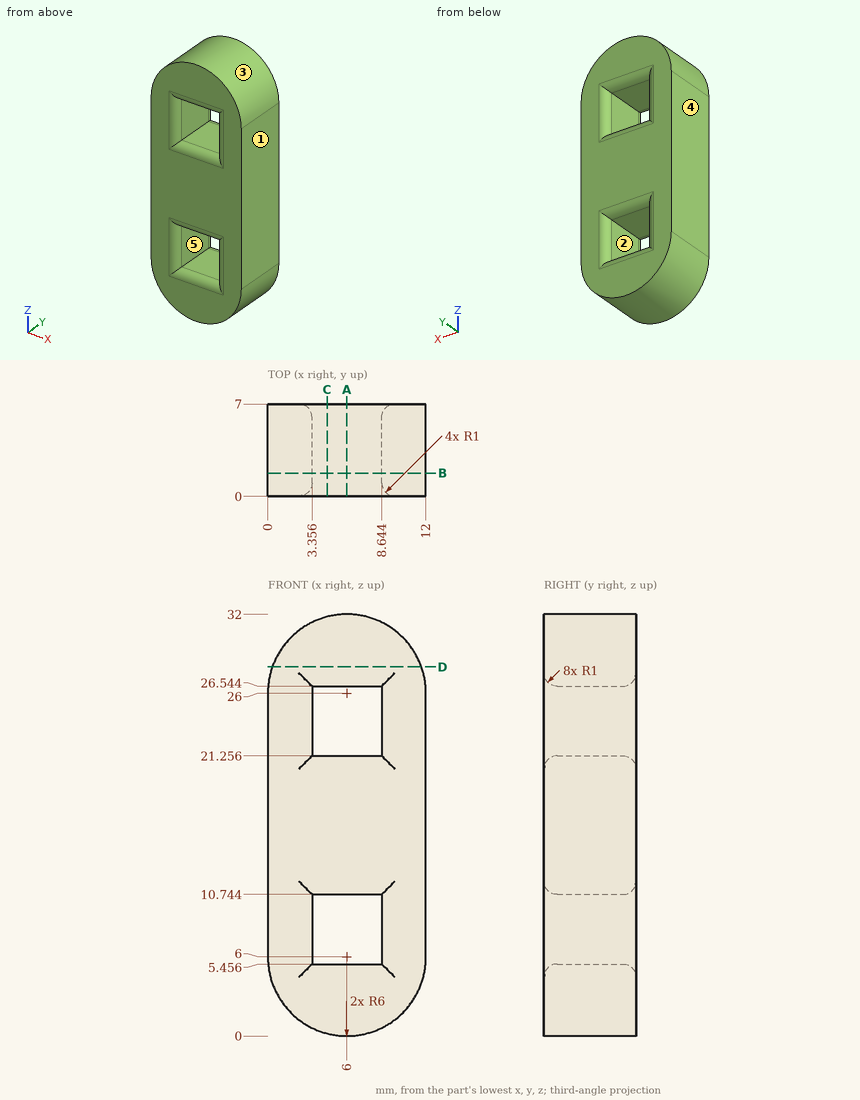
Source: three-view drawing plus pictorial views. Frame: mm from the lowest corner of the part. A direction names the side the tool comes from. Coordinates: 2 decimals unless noted, no trailing zeros. Loops run counter-clockwise (first coordinate to the right, second up) from the corner with the lowest first, then second, coordinate; pieces in that order, holes last. Notation, with made-up numbers: (-30.5, -36.75) -> (-11.5, -36.75) arc R21 ccw to (-11.5, -9.75) -> close; hole circle Ø1 at (-9, 41). An arc over 180 degrees is marked (long way). Answer in a Markdown table with one row per item. Add a question column.
Q1. Section C-C on x = 4.5. Return the cut outline in (y, z).
Q2. Section A-A on x = 6. Return the cut outline in (y, z), and give its area (3 significant figures).
Q3. Section B-B on y = 1.75. Return the cut outline in (x, z), and give its area (3 significant figures).
Q4. Ray query, line 1 along Z through (x, y) = (6.25, 3.25); line 2 along X through (y, z) = (6, 8); line 3 along Z through (x, y) = (6.25, 6.5). Return the intervals inside material, ascending.
Q5. Pull-direction query (Z, two-part tool) for the marked faces 1, 2 and 3; classes: pulls with the +Z half, pulls with the -Z half, needs draft (parallel to the pull), parting line crosses it, or undercut.
Q6. Section D-D on z = 28. Return the cut outline in (x, y), and give its area (3 significant figures).
Q7. Contact query for flat-ended pins moving along their axis: pin 1 Ø1 at (x, y) = (10.5, 1) entering from -Z; pin 2 Ø1 at (y, z) = (4.5, 4) entering from +X; pin 3 Ø2 at (x, z) = (8, 22) entering from -Y (3 decimals). Output: stop coordinate, or through.
Q8. Reachability of the marked faces 4 and 5 from +Z, -Z, +X, -X, +Y, -Y: full face, straight path, thin tool, end or side. Return the list, or none.
Computed values:
| question | item | result |
|---|---|---|
| 1 | outline | (0, 0.19) -> (7, 0.19) -> (7, 4.46) arc R1 ccw to (6, 5.46) -> (1, 5.46) arc R1 ccw to (0, 4.46) -> close; (0, 11.74) arc R1 ccw to (1, 10.74) -> (6, 10.74) arc R1 ccw to (7, 11.74) -> (7, 20.26) arc R1 ccw to (6, 21.26) -> (1, 21.26) arc R1 ccw to (0, 20.26) -> close; (0, 27.54) arc R1 ccw to (1, 26.54) -> (6, 26.54) arc R1 ccw to (7, 27.54) -> (7, 31.81) -> (0, 31.81) -> close |
| 2 | outline | (0, 0) -> (7, 0) -> (7, 4.46) arc R1 ccw to (6, 5.46) -> (1, 5.46) arc R1 ccw to (0, 4.46) -> close; (0, 11.74) arc R1 ccw to (1, 10.74) -> (6, 10.74) arc R1 ccw to (7, 11.74) -> (7, 20.26) arc R1 ccw to (6, 21.26) -> (1, 21.26) arc R1 ccw to (0, 20.26) -> close; (0, 27.54) arc R1 ccw to (1, 26.54) -> (6, 26.54) arc R1 ccw to (7, 27.54) -> (7, 32) -> (0, 32) -> close |
| 2 | area | 148 mm^2 |
| 3 | outline | (0, 6) arc R6 ccw to (12, 6) -> (12, 26) arc R6 ccw to (0, 26) -> close; hole (3.36, 5.46) -> (8.64, 5.46) -> (8.64, 10.74) -> (3.36, 10.74) -> close; hole (3.36, 21.26) -> (8.64, 21.26) -> (8.64, 26.54) -> (3.36, 26.54) -> close |
| 3 | area | 297 mm^2 |
| 4 | line 1 | z = 0.01 to 5.46, 10.74 to 21.26, 26.54 to 31.99 |
| 4 | line 2 | x = 0 to 3.36, 8.64 to 12 |
| 4 | line 3 | z = 0.01 to 5.32, 10.88 to 21.12, 26.68 to 31.99 |
| 5 | face 1 | needs draft |
| 5 | face 2 | undercut |
| 5 | face 3 | pulls with the +Z half |
| 6 | outline | (0.34, 0) -> (11.66, 0) -> (11.66, 7) -> (0.34, 7) -> close |
| 6 | area | 79.2 mm^2 |
| 7 | pin 1 | stops at z = 1.53 |
| 7 | pin 2 | stops at x = 11.81 |
| 7 | pin 3 | stops at y = 0.235 |
| 8 | face 4 | +Z, -Z, -X, +Y, -Y |
| 8 | face 5 | +Y, -Y |
